from build123d import *

# Parameters (mm, degrees)
SKETCH_1_W      = 90
SKETCH_1_H      = 95
EXTRUDE_1_DEPTH = 3
SKETCH_2_W      = 90
SKETCH_2_H      = 95
SKETCH_2_W_2    = 87
SKETCH_2_H_2    = 92
EXTRUDE_2_DEPTH = 60


with BuildPart() as part:
    # 草图1 → 凸台-拉伸1 (new body)
    with BuildSketch(Plane(origin=(0, 0, 0), x_dir=(1, 0, 0), z_dir=(0, 1, 0))):
        Rectangle(SKETCH_1_W, SKETCH_1_H)
    extrude(amount=-EXTRUDE_1_DEPTH)

    # 草图2 → 凸台-拉伸2 (add)
    with BuildSketch(Plane(origin=(0, 0, 0), x_dir=(1, 0, 0), z_dir=(0, 1, 0))):
        Rectangle(SKETCH_2_W, SKETCH_2_H)
        Rectangle(SKETCH_2_W_2, SKETCH_2_H_2, mode=Mode.SUBTRACT)
    extrude(amount=EXTRUDE_2_DEPTH)


solid = part.part
Source: CAD feature listing. Evaluate the final solid. Frame: model axes, mm. A direction names the side the tool comes from. Give positions to 0.01 mm unless a question says otherwise; leave off trailing zeros. Write each loop counter-clockwise with the first axis right and the second up, starting at its lowest first coordinate (ties: lowest second). Pieces come first, ordered by that corner, then holes. Notation, with made-up numbers: M 63.5,39 L 101.5,39 A17 ccw 101.5,67 Z; hole C -12,65 d8. An arc over 180 degrees is marked long. Return JSON: item names as keys, results as strings. Group by question number.
1) Pull-direction query (Z, two-part tool) for faces 1 (the face through (-1, 30, -46)), 2 (the face through (-1, -3, -1)), 3 (the face through (-1, 0, -1)), 4 (the face through (-1, 28, 47.5)); classes: pulls with the +Z half, pulls with the -Z half, needs draft (parallel to the pull), parting line crosses it, or undercut.
2) Cut plane C-C, the plane z = -35. Output: boundary loops of the cut face in (x, y).
3) Cut plane A-A, the plane y = 10.5. Output: boundary loops of the cut face in (x, z), plus the area to 3 significant figures.
4) Set-up query: faces 5 (the face through (-1, 30, 46)), 6 (the face through (-1, 28, -47.5)). Return all of +Z, -Z, +X, -X, +Y, -Y with unobstructed straight access to the full face (end or side cutting, diameter ignored); none if empty.
5) Material intervals for line 1 along Z through (x, y) = (40.5, 46); line 2 along X through (y, z) = (11, -22); line 3 along Y through (x, z) = (-23, -19.5), sorted ascending. Write a range as [from, to].
6) Pin query (flat end, axial travel): P1, Ø1, axis at x = 11, z = -8, coming from the +Y side. Return the tip coordinate at first contact, or that it passes through.
7) Cut plane B-B, the plane x = 31.5. Output: boundary loops of the cut face in (y, z), plus the area to 3 significant figures.
Recorded:
{
 "1": {"face 1": "undercut", "face 2": "needs draft", "face 3": "undercut", "face 4": "pulls with the +Z half"},
 "2": {"outline": "M -45,-3 L 45,-3 L 45,60 L 43.5,60 L 43.5,0 L -43.5,0 L -43.5,60 L -45,60 Z"},
 "3": {"outline": "M -45,-47.5 L 45,-47.5 L 45,47.5 L -45,47.5 Z; hole M -43.5,-46 L 43.5,-46 L 43.5,46 L -43.5,46 Z", "area": "546 mm²"},
 "4": {"face 5": "+Y", "face 6": "-Z, +X, -X, +Y, -Y"},
 "5": {"line 1": "z = [-47.5, -46], [46, 47.5]", "line 2": "x = [-45, -43.5], [43.5, 45]", "line 3": "y = [-3, 0]"},
 "6": {"P1": "stops at y = 0"},
 "7": {"outline": "M -3,-47.5 L 60,-47.5 L 60,-46 L 0,-46 L 0,46 L 60,46 L 60,47.5 L -3,47.5 Z", "area": "465 mm²"}
}
